from build123d import *

# Parameters (mm, degrees)
F0_R     = 13.75
F0_R_2   = 11.5
F1_DEPTH = 8.4
F3_R     = 11.5
F4_DEPTH = 4
F6_SIZE  = 2
F7_SIZE  = 0.99999


# Not quite as in the source:
# - a fillet or chamfer that OpenCascade refuses, or shapes differently, is made with other operations: its cross-section is extruded or revolved along the edge and cut away or added
# - a fillet or chamfer is up to 0.001 mm smaller than in the source, because OpenCascade refuses the exact size


with BuildPart() as f1:
    # F0 (on Top) → F1 (new body)
    with BuildSketch(Plane.XY):
        Circle(F0_R)
        Circle(F0_R_2, mode=Mode.SUBTRACT)
    extrude(amount=F1_DEPTH)

    # F3 (on offset) → F4 (join)
    with BuildSketch(Plane.XY.offset(5.5)):
        with BuildLine():
            ThreePointArc((-16.75, 0), (-11.8440385849, -11.8440385849), (0, -16.75))
            ThreePointArc((0, -16.75), (11.8440385849, -11.8440385849), (16.75, 0))
            ThreePointArc((16.75, 0), (11.8440385849, 11.8440385849), (0, 16.75))
            ThreePointArc((0, 16.75), (-11.8440385849, 11.8440385849), (-16.75, 0))
        make_face()
        Circle(F3_R, mode=Mode.SUBTRACT)
    extrude(amount=F4_DEPTH)

    # F5: chamfer of 2 x 5.4949548389 on 1 edges, made by hand

    # F5_s1 → F5_t2 (revolve, cut)
    with BuildSketch(Plane.XZ):
        Polygon((16.9949548389, 9.5), (11.5, 7.5), (11.5, 9.5), align=None)
    revolve(axis=Axis((0, 0, 9.5), (0, 0, 1)), mode=Mode.SUBTRACT)

    # F6
    f6_edges = [f1.edges().sort_by_distance(p)[0] for p in [
        (-13.75, 0, 5.5),
    ]]
    chamfer(f6_edges, length=F6_SIZE)

    # F7 (size 1 in the source; OpenCascade refuses exactly that, so slightly less here)
    f7_edges = [f1.edges().sort_by_distance(p)[0] for p in [
        (0, 16.75, 5.5),
    ]]
    chamfer(f7_edges, length=F7_SIZE)


solid = f1.part
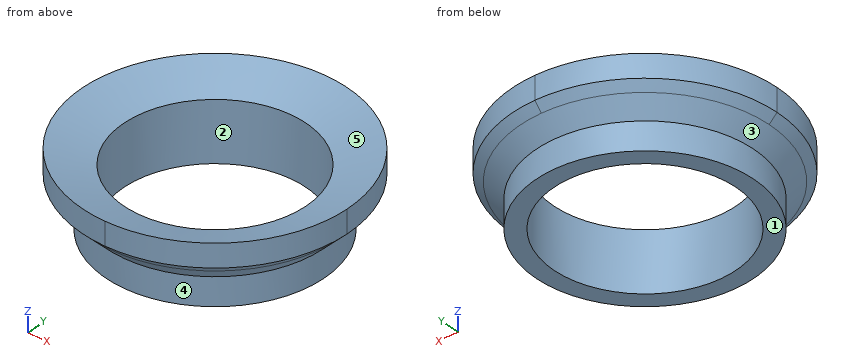
Can you work these out from the model? Positions are in its coordinate system, mm. Face numbers are marked on the shaded views. A direction names the side the tool comes from. Round coordinates to 2 decimals unless told otherwise and drop trailing zeros. Order: outer loops, then holes, each group sorted by start corner. A loop starts at its lowest first (then second) coordinate and runs counter-clockwise, first axis right, second up. Notation, with made-up numbers: M 72.25,88.5 L 106.25,88.5 A32 ccw 106.25,120.5 Z; hole C 53,23 d7. An arc over 180 degrees is marked long. Use a Markdown table: item, result.
1) I'm going to push flat-ended pins straight in: P1, Ø3, axis at x = 2.5, z = 3.5, coming from the +Y side; P2, Ø8, axis at x = -3, y = -8, coming from the +Z side; P3, Ø1, axis at x = -8.5, y = -9.5, coming from the +Z side. Where does each tip first touch, or does it pass through?
Geometry says:
| item | result |
|---|---|
| P1 | stops at y = 15.06 |
| P2 | stops at z = 7.88 |
| P3 | stops at z = 8.14 |
2) On a 3-axis mill with a long thin cutter (end or side, diameter ignored), from which of +Z, -Z, +X, -X, +Y, -Y can I reach the whole of each face in a straight line? I mean the marked faces 4 and 5. Say none if no direction works.
Geometry says:
| item | result |
|---|---|
| face 4 | -Z |
| face 5 | +Z |
3) Imagine slicing it at B-B (z = 4.25). List the corners of the cut face in (x, y) for me.
Geometry says:
| item | result |
|---|---|
| outline | C 0,0 d29; hole C 0,0 d23 |
4) If I drill on line 1 along Y through (x, z) = (0, 3); line 2 along Y through (x, z) = (0, 5.5); line 3 along X through (y, z) = (4.5, 4), over which ranges is the centre line in solid material (lowest first)?
Geometry says:
| item | result |
|---|---|
| line 1 | y = -13.75 to -11.5, 11.5 to 13.75 |
| line 2 | y = -15.75 to -11.5, 11.5 to 15.75 |
| line 3 | x = -13.52 to -10.58, 10.58 to 13.52 |
5) Imagine slicing it at A-A (z = 2). List the corners of the cut face in (x, y) for me.
Geometry says:
| item | result |
|---|---|
| outline | C 0,0 d27.5; hole C 0,0 d23 |
6) If we mould it in two halves opening along Y, with no side actions, what happens to the marked faces 1, 2 and 3? For each: +Y half, -Y half, draft (parallel to the pull), parting line (faces both ways), or undercut.
Geometry says:
| item | result |
|---|---|
| face 1 | draft |
| face 2 | undercut |
| face 3 | parting line |
